from build123d import *

# Parameters (mm, degrees)
SKETCH4_R            = 59
BOSS_EXTRUDE3_DEPTH  = 2
SKETCH5_R            = 1.375
BOSS_EXTRUDE5_DEPTH  = 7
SKETCH8_R            = 2.375
BOSS_EXTRUDE6_DEPTH  = 2
BOSS_EXTRUDE7_DEPTH  = 18
SKETCH10_R           = 7.5
CUT_EXTRUDE1_DEPTH   = 18
SKETCH12_R           = 57.5
CUT_EXTRUDE2_DEPTH   = 5
CUT_EXTRUDE3_DEPTH   = 5.5
SKETCH14_R           = 44.428135616
CUT_EXTRUDE4_DEPTH   = 32
BOSS_EXTRUDE8_DEPTH  = 3
BOSS_EXTRUDE9_DEPTH  = 2
SKETCH18_W           = 40
SKETCH18_H           = 24
CUT_EXTRUDE5_DEPTH   = 2
SKETCH19_W           = 4
SKETCH19_H           = 6
SKETCH19_W_2         = 8
SKETCH19_H_2         = 24
BOSS_EXTRUDE10_DEPTH = 2
SKETCH20_R           = 71.034408428
SKETCH20_R_2         = 50.972397724
CUT_EXTRUDE6_DEPTH   = 57
SKETCH21_R           = 79.144233261
SKETCH21_R_2         = 57
CUT_EXTRUDE8_DEPTH   = 57
BOSS_EXTRUDE11_DEPTH = 22
SKETCH24_R           = 89.588110905
SKETCH24_R_2         = 57
CUT_EXTRUDE12_DEPTH  = 75
SKETCH25_R           = 63.08525578
SKETCH25_R_2         = 55
CUT_EXTRUDE13_DEPTH  = 10
SKETCH26_R           = 62.71577626
SKETCH26_R_2         = 55
CUT_EXTRUDE14_DEPTH  = 43
SKETCH27_R           = 8.628716001
SKETCH27_R_2         = 7.77122145
SKETCH27_R_3         = 11.532169803
SKETCH27_R_4         = 7.052668864
CUT_EXTRUDE15_DEPTH  = 22
SKETCH28_R           = 55
BOSS_EXTRUDE12_DEPTH = 2
SKETCH29_W           = 5
SKETCH29_H           = 12
CUT_EXTRUDE16_DEPTH  = 3
SKETCH30_R           = 6.25
CUT_EXTRUDE17_DEPTH  = 3
SKETCH31_W           = 50
SKETCH31_H           = 10
CUT_EXTRUDE18_DEPTH  = 3


with BuildPart() as part:
    # Sketch4 → Boss-Extrude3 (new body)
    with BuildSketch(Plane.XY):
        Circle(SKETCH4_R)
    extrude(amount=BOSS_EXTRUDE3_DEPTH)

    # Sketch5 → Boss-Extrude5 (add)
    with BuildSketch(Plane.XY.offset(2)):
        with Locations((-22.5, 27.5)):
            Circle(SKETCH5_R)
        with Locations((22.5, 27.5)):
            Circle(SKETCH5_R)
        with Locations((22.5, -27.5)):
            Circle(SKETCH5_R)
        with Locations((-22.5, -27.5)):
            Circle(SKETCH5_R)
    extrude(amount=BOSS_EXTRUDE5_DEPTH)

    # Sketch8 → Boss-Extrude6 (add)
    with BuildSketch(Plane.XY.offset(2)):
        with Locations((-22.5, 27.5)):
            Circle(SKETCH8_R)
        with Locations((22.5, 27.5)):
            Circle(SKETCH8_R)
        with Locations((-22.5, -27.5)):
            Circle(SKETCH8_R)
        with Locations((22.5, -27.5)):
            Circle(SKETCH8_R)
    extrude(amount=BOSS_EXTRUDE6_DEPTH)

    # Sketch9 → Boss-Extrude7 (add)
    with BuildSketch(Plane.XY.offset(2)):
        with BuildLine():
            ThreePointArc((-4.745762712, 55.798546005), (0, 56), (4.745762712, 55.798546005))
            Line((4.745762712, 55.798546005), (5, 58.787753827))
            ThreePointArc((5, 58.787753827), (0, 59), (-5, 58.787753827))
            Line((-5, 58.787753827), (-4.745762712, 55.798546005))
        make_face()
        with BuildLine():
            Line((-55.798546005, 4.745762712), (-58.787753827, 5))
            ThreePointArc((-58.787753827, 5), (-59, 0), (-58.787753827, -5))
            Line((-58.787753827, -5), (-55.798546005, -4.745762712))
            ThreePointArc((-55.798546005, -4.745762712), (-56, 0), (-55.798546005, 4.745762712))
        make_face()
        with BuildLine():
            ThreePointArc((58.787753827, -5), (59, 0), (58.787753827, 5))
            Line((58.787753827, 5), (55.798546005, 4.745762712))
            ThreePointArc((55.798546005, 4.745762712), (56, 0), (55.798546005, -4.745762712))
            Line((55.798546005, -4.745762712), (58.787753827, -5))
        make_face()
        with BuildLine():
            ThreePointArc((-4.745762712, -55.798546005), (0, -56), (4.745762712, -55.798546005))
            Line((4.745762712, -55.798546005), (5, -58.787753827))
            ThreePointArc((5, -58.787753827), (0, -59), (-5, -58.787753827))
            Line((-5, -58.787753827), (-4.745762712, -55.798546005))
        make_face()
    extrude(amount=BOSS_EXTRUDE7_DEPTH)

    # Sketch10 → Cut-Extrude1 (cut)
    with BuildSketch(Plane.XY.offset(2)):
        with Locations((-40, 0)):
            Circle(SKETCH10_R)
    extrude(amount=-CUT_EXTRUDE1_DEPTH, mode=Mode.SUBTRACT)

    # Sketch12 → Cut-Extrude2 (cut)
    with BuildSketch(Plane.XY.offset(20)):
        Circle(SKETCH12_R)
    extrude(amount=-CUT_EXTRUDE2_DEPTH, mode=Mode.SUBTRACT)

    # Sketch13 → Cut-Extrude3 (cut)
    with BuildSketch(Plane(origin=(0, 0, 0), x_dir=(-1, 0, 0), z_dir=(0, 0, -1))):
        with BuildLine():
            Line((-57.243329786, 4.868644068), (-58.787753827, 5))
            ThreePointArc((-58.787753827, 5), (-59, 0), (-58.787753827, -5))
            Line((-58.787753827, -5), (-57.243329786, -4.868644068))
            ThreePointArc((-57.243329786, -4.868644068), (-57.45, 0), (-57.243329786, 4.868644068))
        make_face()
        with BuildLine():
            ThreePointArc((5, 58.787753827), (0, 59), (-5, 58.787753827))
            Line((-5, 58.787753827), (-4.868644068, 57.243329786))
            ThreePointArc((-4.868644068, 57.243329786), (0, 57.45), (4.868644068, 57.243329786))
            Line((4.868644068, 57.243329786), (5, 58.787753827))
        make_face()
        with BuildLine():
            Line((-4.868644068, -57.243329786), (-5, -58.787753827))
            ThreePointArc((-5, -58.787753827), (0, -59), (5, -58.787753827))
            Line((5, -58.787753827), (4.868644068, -57.243329786))
            ThreePointArc((4.868644068, -57.243329786), (0, -57.45), (-4.868644068, -57.243329786))
        make_face()
        with BuildLine():
            ThreePointArc((58.787753827, -5), (59, 0), (58.787753827, 5))
            Line((58.787753827, 5), (57.243329786, 4.868644068))
            ThreePointArc((57.243329786, 4.868644068), (57.45, 0), (57.243329786, -4.868644068))
            Line((57.243329786, -4.868644068), (58.787753827, -5))
        make_face()
    extrude(amount=-CUT_EXTRUDE3_DEPTH, mode=Mode.SUBTRACT)

    # Sketch14 → Cut-Extrude4 (cut)
    with BuildSketch(Plane.XY.offset(2)):
        Circle(SKETCH14_R)
    extrude(amount=CUT_EXTRUDE4_DEPTH, mode=Mode.SUBTRACT)

    # Sketch15 → Boss-Extrude8 (add)
    with BuildSketch(Plane.XY.offset(2)):
        Polygon((21.5, -6), (21.5, 6), (-24.5, 6), (-24.5, 12), (24.5, 12), (24.5, -12), (-24.5, -12), (-24.5, -6), align=None)
    extrude(amount=BOSS_EXTRUDE8_DEPTH)

    # Sketch17 → Boss-Extrude9 (add)
    with BuildSketch(Plane.XY.offset(5)):
        Polygon((21.5, -9), (-21.5, -9), (-24.5, -9), (-24.5, -12), (24.5, -12), (24.5, 12), (-24.5, 12), (-24.5, 9), (-21.5, 9), (21.5, 9), align=None)
    extrude(amount=BOSS_EXTRUDE9_DEPTH)

    # Sketch18 → Cut-Extrude5 (cut)
    with BuildSketch(Plane.XY.offset(7)):
        with Locations((-0.5, 0)):
            Rectangle(SKETCH18_W, SKETCH18_H)
    extrude(amount=-CUT_EXTRUDE5_DEPTH, mode=Mode.SUBTRACT)

    # Sketch19 → Boss-Extrude10 (add)
    with BuildSketch(Plane.XY.offset(7)):
        with Locations((-22.5, 9)):
            Rectangle(SKETCH19_W, SKETCH19_H)
        with Locations((-22.5, -9)):
            Rectangle(SKETCH19_W, SKETCH19_H)
        with Locations((20.5, 0)):
            Rectangle(SKETCH19_W_2, SKETCH19_H_2)
    extrude(amount=BOSS_EXTRUDE10_DEPTH)

    # Sketch20 → Cut-Extrude6 (cut)
    with BuildSketch(Plane.XY.offset(2)):
        Circle(SKETCH20_R)
        Circle(SKETCH20_R_2, mode=Mode.SUBTRACT)
    extrude(amount=CUT_EXTRUDE6_DEPTH, mode=Mode.SUBTRACT)

    # Sketch21 → Cut-Extrude8 (cut)
    with BuildSketch(Plane.XY.offset(2)):
        Circle(SKETCH21_R)
        Circle(SKETCH21_R_2, mode=Mode.SUBTRACT)
    extrude(amount=-CUT_EXTRUDE8_DEPTH, mode=Mode.SUBTRACT)

    # Sketch23 → Boss-Extrude11 (add)
    with BuildSketch(Plane.XY.offset(2)):
        with BuildLine():
            ThreePointArc((4.98087362, 56.781959265), (2.492821884, 56.945463727), (0, 57))
            ThreePointArc((0, 57), (-2.492821884, 56.945463727), (-4.98087362, 56.781959265))
            Line((-4.98087362, 56.781959265), (-4.631338629, 52.797260369))
            ThreePointArc((-4.631338629, 52.797260369), (0, 53), (4.631338629, 52.797260369))
            Line((4.631338629, 52.797260369), (4.98087362, 56.781959265))
        make_face()
        with BuildLine():
            ThreePointArc((57, 0), (56.945463727, 2.492821884), (56.781959265, 4.98087362))
            Line((56.781959265, 4.98087362), (52.797260369, 4.631338629))
            ThreePointArc((52.797260369, 4.631338629), (53, 0), (52.797260369, -4.631338629))
            Line((52.797260369, -4.631338629), (56.781959265, -4.98087362))
            ThreePointArc((56.781959265, -4.98087362), (56.945463727, -2.492821884), (57, 0))
        make_face()
        with BuildLine():
            ThreePointArc((-52.797260369, 4.631338629), (-53, 0), (-52.797260369, -4.631338629))
            Line((-52.797260369, -4.631338629), (-57, -5))
            Line((-57, -5), (-57, 5))
            Line((-57, 5), (-52.797260369, 4.631338629))
        make_face()
        with BuildLine():
            ThreePointArc((-4.631338629, -52.797260369), (0, -53), (4.631338629, -52.797260369))
            Line((4.631338629, -52.797260369), (5, -57))
            Line((5, -57), (-5, -57))
            Line((-5, -57), (-4.631338629, -52.797260369))
        make_face()
    extrude(amount=BOSS_EXTRUDE11_DEPTH)

    # Sketch24 → Cut-Extrude12 (cut)
    with BuildSketch(Plane.XY.offset(24)):
        Circle(SKETCH24_R)
        Circle(SKETCH24_R_2, mode=Mode.SUBTRACT)
    extrude(amount=-CUT_EXTRUDE12_DEPTH, mode=Mode.SUBTRACT)

    # Sketch25 → Cut-Extrude13 (cut)
    with BuildSketch(Plane.XY.offset(2)):
        Circle(SKETCH25_R)
        Circle(SKETCH25_R_2, mode=Mode.SUBTRACT)
    extrude(amount=-CUT_EXTRUDE13_DEPTH, mode=Mode.SUBTRACT)

    # Sketch26 → Cut-Extrude14 (cut)
    with BuildSketch(Plane(origin=(0, 0, 0), x_dir=(-1, 0, 0), z_dir=(0, 0, -1))):
        Circle(SKETCH26_R)
        Circle(SKETCH26_R_2, mode=Mode.SUBTRACT)
    extrude(amount=-CUT_EXTRUDE14_DEPTH, mode=Mode.SUBTRACT)

    # Sketch27 → Cut-Extrude15 (cut)
    with BuildSketch(Plane.XY.offset(24)):
        with Locations((-55, 0)):
            Circle(SKETCH27_R)
        with Locations((0, -55)):
            Circle(SKETCH27_R_2)
        with Locations((55, 0)):
            Circle(SKETCH27_R_3)
        with Locations((0, 53)):
            Circle(SKETCH27_R_4)
    extrude(amount=-CUT_EXTRUDE15_DEPTH, mode=Mode.SUBTRACT)

    # Sketch28 → Boss-Extrude12 (add)
    with BuildSketch(Plane.XY.offset(2)):
        Circle(SKETCH28_R)
    extrude(amount=-BOSS_EXTRUDE12_DEPTH)

    # Sketch29 → Cut-Extrude16 (cut)
    with BuildSketch(Plane.XY.offset(9)):
        with Locations((19, 0)):
            Rectangle(SKETCH29_W, SKETCH29_H)
    extrude(amount=-CUT_EXTRUDE16_DEPTH, mode=Mode.SUBTRACT)

    # Sketch30 → Cut-Extrude17 (cut)
    with BuildSketch(Plane.XY.offset(2)):
        with Locations((0, 44.5)):
            Circle(SKETCH30_R)
        with Locations((44.5, 0)):
            Circle(SKETCH30_R)
        with Locations((0, -44.5)):
            Circle(SKETCH30_R)
        with Locations((-44.5, 0)):
            Circle(SKETCH30_R)
    extrude(amount=-CUT_EXTRUDE17_DEPTH, mode=Mode.SUBTRACT)

    # Sketch31 → Cut-Extrude18 (cut)
    with BuildSketch(Plane.XY.offset(2)):
        with Locations((0, 30)):
            Rectangle(SKETCH31_W, SKETCH31_H)
        with Locations((0, -30)):
            Rectangle(SKETCH31_W, SKETCH31_H)
    extrude(amount=-CUT_EXTRUDE18_DEPTH, mode=Mode.SUBTRACT)


solid = part.part
Geometry check sheet. Reference: the model listing, model coordinates, mm. A direction names the side the tool comes from. Coordinates: 2 decimals unless noted, no trailing zeros. Order: outer loops, then holes, each group sorted by start corner. A loop starts at its lowest first (then second) coordinate and runs counter-clockwise, first axis right, second up. Notation, with made-up numbers: (89.25, 19) - (106.25, 19) arc R11 ccw to (106.25, 25) - close; hole circle Ø10 at (73, 17.25). An arc over 180 degrees is marked (long way). One line per item, written item: value.
(1) Release check for a two-part mould opening along Z. For faces 5 (the face through (-23, 9, 9)), 6 (the face through (18, 8, 7)), 7 (the face through (-1, 1, 0)) record: +Z half, -Z half, draft (parallel to the pull), parting line (faces both ways), or undercut.
Data:
face 5: +Z half
face 6: undercut
face 7: -Z half
(2) Thickness scan on probe 1 along Y at (x, z) = (0, 1.55); probe 2 along Y at (x, z) = (18, 7.25); probe 3 along X at (y, z) = (-5.5, 1). Record the ranges inside material, lowest first. Write a range as from..to.
Data:
probe 1: y = -55..-50.75, -38.25..-35, -25..25, 35..38.25, 50.75..55
probe 2: y = -12..-6, 6..12
probe 3: x = -54.72..-47.47, -41.53..41.53, 47.47..54.72
(3) Sectioned sample at A-A (y = 0). Enter the section's corners in (x, z).
Data:
outline: (-55, 0) - (-50.75, 0) - (-50.75, 2) - (-55, 2) - close; (-38.25, 0) - (38.25, 0) - (38.25, 2) - (24.5, 2) - (24.5, 9) - (21.5, 9) - (21.5, 2) - (-38.25, 2) - close; (50.75, 0) - (55, 0) - (55, 2) - (50.75, 2) - close
(4) Depth check by flat-ended pin: pin 1 Ø12 at (x, y) = (24, -32) entering from +Z; pin 2 Ø5 at (y, z) = (40, 2.5) entering from +X; pin 3 Ø2 at (y, z) = (27.5, 1) entering from +X; pin 4 Ø7.5 at (x, y) = (-44.5, 0) entering from -Z. Enter the tip coordinate at first touch or a pass-through.
Data:
pin 1: stops at z = 2
pin 2: stops at x = 40.19
pin 3: stops at x = 48.19
pin 4: passes through
(5) Sectioned sample at C-C (x = 44.5). Enter the section's corners in (y, z).
Data:
outline: (-32.32, 0) - (-6.25, 0) - (-6.25, 2) - (-32.32, 2) - close; (6.25, 0) - (32.32, 0) - (32.32, 2) - (6.25, 2) - close
(6) Sectioned sample at B-B (x = 0). Enter the section's corners in (y, z), and give its area (3 significant figures).
Data:
outline: (-55, 0) - (-50.75, 0) - (-50.75, 2) - (-55, 2) - close; (-38.25, 0) - (-35, 0) - (-35, 2) - (-38.25, 2) - close; (-25, 0) - (25, 0) - (25, 2) - (12, 2) - (12, 5) - (6, 5) - (6, 2) - (-6, 2) - (-6, 5) - (-12, 5) - (-12, 2) - (-25, 2) - close; (35, 0) - (38.25, 0) - (38.25, 2) - (35, 2) - close; (50.75, 0) - (55, 0) - (55, 2) - (50.75, 2) - close
area: 166 mm^2
(7) Access from +Z, -Z, +X, -X, +Y, -Y to the whole of each face (thin tool, end or side, straight path). Record for faces 1 (the face through (18, -8, 7)), 2 (the face through (-2, -6, 3)), 3 (the face through (0, -12, 4)), 4 (the face through (0, 12, 4)).
Data:
face 1: none
face 2: +Z, -X
face 3: +Z, +X, -X, -Y
face 4: +Z, +X, -X, +Y
